Input: part model. Units: mm. Frame: model coordinates. Face numbers are marked on the shaded views. Give positions to 0.01 mm unless a question says otherwise; leave off trailing zeros. Loops run counter-clockwise (first coordinate to the right, second up) from the corner with the lowest first, then second, coordinate; pieces in that order, holes last. Notation, with made-up numbers: M 19,66 L 23,66 A24 cw 23,80 Z; hole C 48.5,64 d9. An arc over 180 degrees is marked long. Answer as a JSON object with one key per item and string values. Group by question number.
1) Ray query, L1, parallel to Z at x = 1, y = 0; L2, parallel to Y at x = -1, z = 10.25; L3, parallel to Y at x = -1, z = 10.5. Return the intervals inside material, ascending.
2) Draft query along X for the marked faces 1, 2, 3 and 4. Return one class per face: +X half, -X half, draft (parallel to the pull), parting line (faces both ways), or undercut.
3) First-contact query: P1, Ø1.4, axis at y = -0.5, z = 10.5, coming from the +X side; P2, Ø1.9, axis at y = 0, z = 10, coming from the -X side; P3, Ø3, axis at x = -2.5, z = 3.5, coming from the +Y side. Flat tips, straight axial feed; report the tip coordinate or a pass-through.
4) Section query A-A on z = 7.5. Return loops of the section in (x, y), plus the area to 3 significant figures.
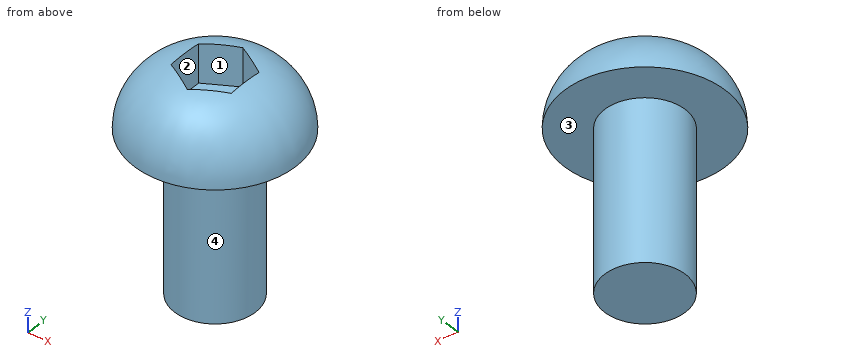
Autodesk Inventor part; units mm, degrees
ref_plane "YZ Plane" through (0, 0, 0) normal (1, 0, 0) x (0, 1, 0)
ref_plane "XZ Plane" through (0, 0, 0) normal (0, 1, 0) x (-1, 0, 0)
ref_plane "XY Plane" through (0, 0, 0) normal (0, 0, 1) x (1, 0, 0)
sketch "スケッチ1" plane through (0, 0, 0) normal (0, 0, 1) x (1, 0, 0)
  circle A0 centre (0, 0) radius 2
  dimension "d0" = 4
extrude "押し出し1" add sketch "スケッチ1" along normal blind 8
sketch "スケッチ2" plane through (0, 0, 8) normal (0, 0, 1) x (1, 0, 0)
  circle A0 centre (0, 0) radius 2
  circle A1 centre (0, 0) radius 4
  dimension "d3" = 8
extrude "押し出し2" add sketch "スケッチ2" along normal blind 3 contours A0 | A1
fillet "フィレット1" radius 3 1 edges at (-4, 0, 11)
thread "ねじ1"
sketch "スケッチ3" plane through (0, 0, 11) normal (0, 0, 1) x (1, 0, 0)
  line L0 (-1.5, 0.866) -> (0, 1.7321)
  line L1 (0, 1.7321) -> (1.5, 0.866)
  line L2 (1.5, 0.866) -> (1.5, -0.866)
  line L3 (1.5, -0.866) -> (0, -1.7321)
  line L4 (0, -1.7321) -> (-1.5, -0.866)
  line L5 (-1.5, -0.866) -> (-1.5, 0.866)
  point P0 (0, 0)
  point P1 (0, 0)
  point P2 (-1.5, 0)
  dimension "d9" = 3
extrude "押し出し3" cut sketch "スケッチ3" against normal blind 2
properties part number "SB　M4 8mm なべネジ" material "Stainless Steel, 440C"
Output:
{
 "1": {"L1": "z = 0 to 9", "L2": "y = -2.81 to -1.15, 1.15 to 2.81", "L3": "y = -2.46 to -1.15, 1.15 to 2.46"},
 "2": {"face 1": "undercut", "face 2": "undercut", "face 3": "draft", "face 4": "parting line"},
 "3": {"P1": "stops at x = 3.37", "P2": "stops at x = -3.81", "P3": "stops at y = 1.73"},
 "4": {"outline": "C 0,0 d4", "area": "12.6 mm^2"}
}
